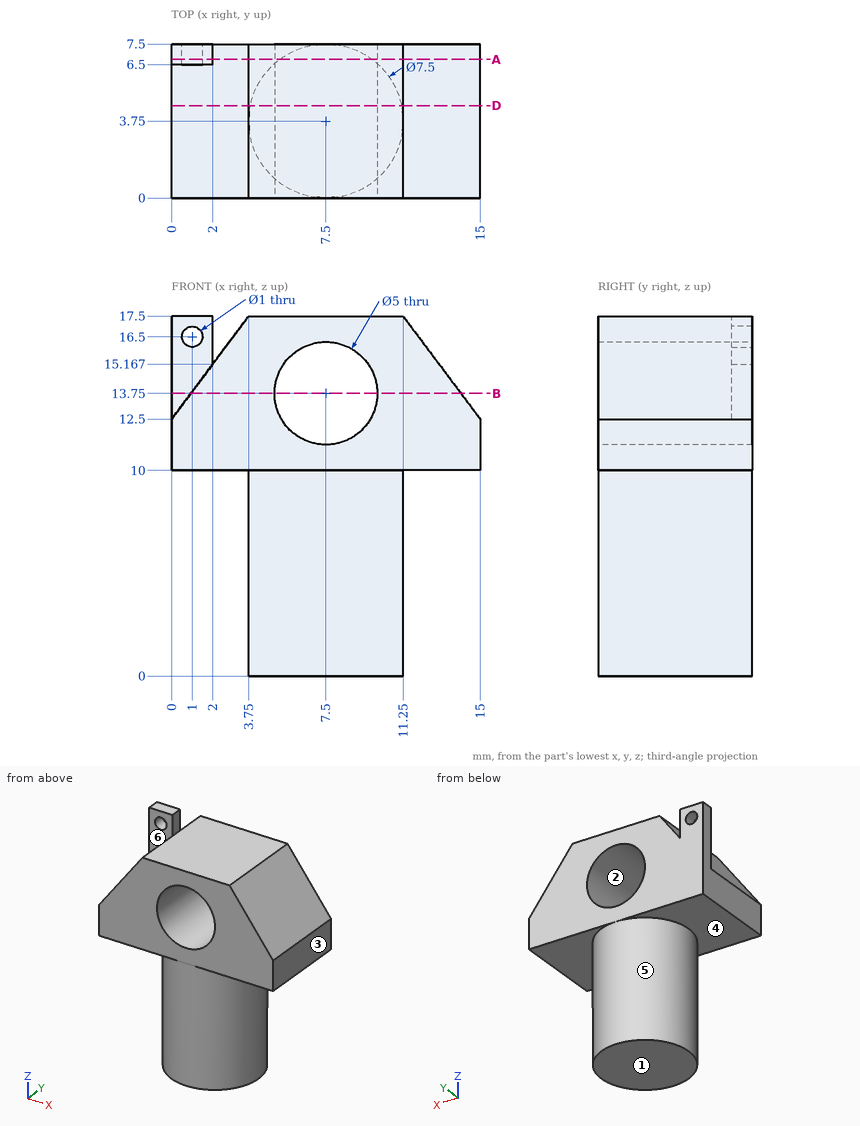
Check sheet for the drawn part. Datum: minimum x, y, z corner. Units: mm. A direction names the side the tool comes from. Coordinates: 2 decimals unless noted, no trailing zeros. Write each loop counter-clockwise with the first axis right and the second up, starting at its lowest first coordinate (ties: lowest second). Pieces come first, ordered by that corner, then holes. Notation, with made-up numbers: M 43,25 L 102,25 A15 cw 102,30 Z; hole C 59.5,23 d9. An arc over 180 degrees is marked long. One line per item, written item: value.
Item 1: Section check A-A, the plane y = 6.75. Record the boundary of the cut face in (x, z).
Check sheet entries:
outline: M 0,10 L 5.25,10 L 5.25,0 L 9.75,0 L 9.75,10 L 15,10 L 15,12.5 L 11.25,17.5 L 3.75,17.5 L 2,15.17 L 2,17.5 L 0,17.5 Z; hole C 1,16.5 d1; hole C 7.5,13.75 d5
Item 2: Scan lines: line 1 along Z through (x, y) = (1, 6.75); line 2 along Z through (x, y) = (7.5, 2.5); line 3 along Z through (x, y) = (2, 4.5) (1 decimal). Record each from-to range of solid material in increasing order.
Check sheet entries:
line 1: z = 10 to 16, 17 to 17.5
line 2: z = 0 to 11.25, 16.25 to 17.5
line 3: z = 10 to 15.2
Item 3: Gauge pin test, flat ends, axial feed: pin 1 Ø3 at (x, y) = (2.5, 1) entering from -Z; pin 2 Ø1 at (y, z) = (4.5, 15.5) entering from +X (1 decimal); pin 3 Ø3 at (x, z) = (7.5, 13.75) entering from +Y; pin 4 Ø0.8 at (y, z) = (7, 16) entering from +X (1 decimal). Record the tip position at first contact, or that the pin passes through.
Check sheet entries:
pin 1: stops at z = 10
pin 2: stops at x = 13.1
pin 3: passes through
pin 4: stops at x = 12.7
Item 4: Section check B-B, the plane z = 13.75. Record the boundary of the cut face in (x, y).
Check sheet entries:
outline: M 0,6.5 L 0.94,6.5 L 0.94,0 L 5,0 L 5,7.5 L 0,7.5 Z; M 10,0 L 14.06,0 L 14.06,7.5 L 10,7.5 Z
Item 5: Section check D-D, the plane y = 4.5. Record the boundary of the cut face in (x, z).
Check sheet entries:
outline: M 0,10 L 3.83,10 L 3.83,0 L 11.17,0 L 11.17,10 L 15,10 L 15,12.5 L 11.25,17.5 L 3.75,17.5 L 0,12.5 Z; hole C 7.5,13.75 d5
Item 6: Mould release check, pull along Z, two halves, no side actions. Record for the marked faces 1, 2 and 3: pulls with the +Z half, pulls with the -Z half, needs draft (parallel to the pull), parting line crosses it, or undercut.
Check sheet entries:
face 1: pulls with the -Z half
face 2: undercut
face 3: needs draft
Item 7: Access from +Z, -Z, +X, -X, +Y, -Y to the whole of each face (thin tool, end or side, straight path). Record for the marked faces 4, 5 and 6.
Check sheet entries:
face 4: -Z, -X
face 5: -Z
face 6: +Z, -X, -Y
